Design review of the part shown in the three views and the two pictorial views. Dimensions are in mm from the part's minimum x, y and z. Give positions to 0.01 mm unless a question says otherwise; leave off trailing zeros. Loops run counter-clockwise (first coordinate to the right, second up) from the corner with the lowest first, then second, coordinate; pieces in that order, holes last. Notation, with made-up numbers: (-20, 11) -> (29, 11) arc R19 cw to (29, 48) -> close; hole circle Ø5 at (-30, 6). An arc over 180 degrees is marked (long way). Answer as CSV lines item,"result".
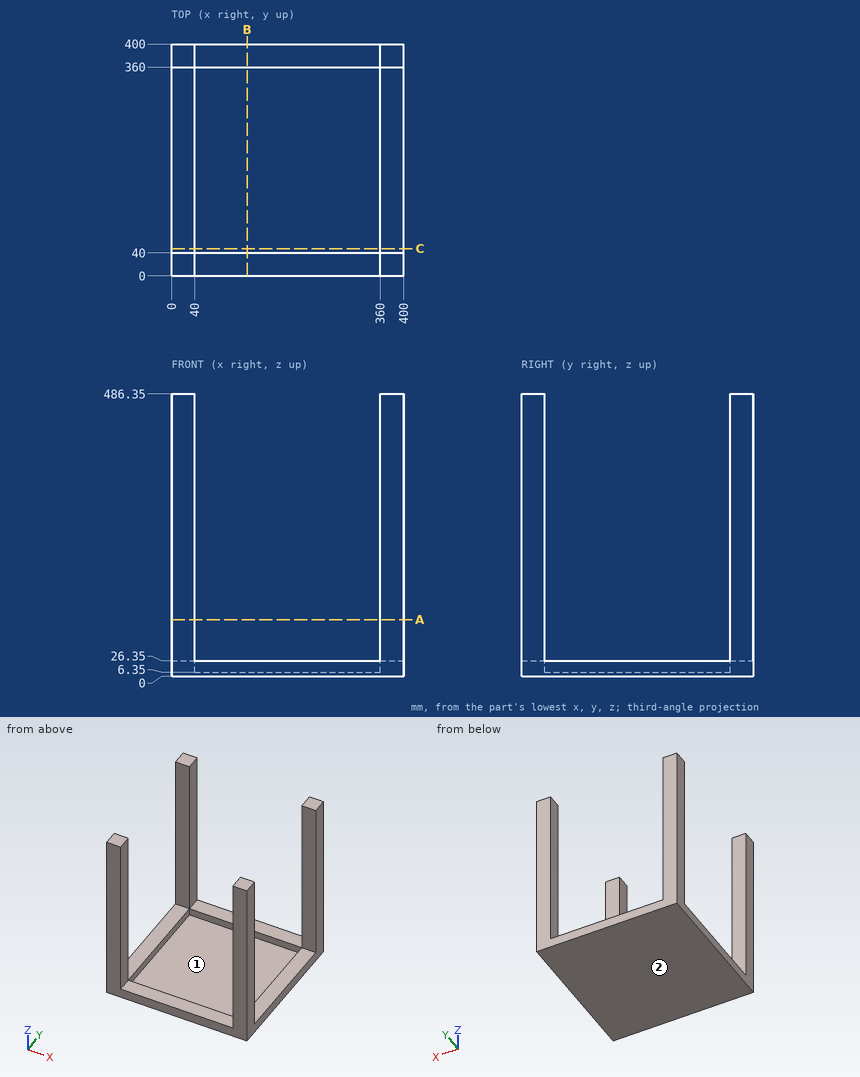
Q1. We need section A-A, the plane z = 97. State the section outline as (x, y) points.
Filled sheet:
outline,"(0, 0) -> (40, 0) -> (40, 40) -> (0, 40) -> close; (0, 360) -> (40, 360) -> (40, 400) -> (0, 400) -> close; (360, 0) -> (400, 0) -> (400, 40) -> (360, 40) -> close; (360, 360) -> (400, 360) -> (400, 400) -> (360, 400) -> close"
Q2. Clearance check with a flat-ended pin moving along its axis: pin 1 Ø8 at (x, y) = (143, 346.5) entering from +Z. State where the tip first meets the part, or that it passes through.
Filled sheet:
pin 1,"stops at z = 6.35"
Q3. To check wall thickness, follow probe 1 along Y at (x, z) = (38.5, 199); probe 2 along Z at (x, y) = (50.5, 90). State the ranges of each line that lie inside material, in increasing order. Write a range as from..to.
Filled sheet:
probe 1,"y = 0..40, 360..400"
probe 2,"z = 0..6.35"
Q4. The part is to be moulded in two halves that separate along Y. For the marked faces 1 and 2, say which applies: pulls with the +Y half, pulls with the -Y half, needs draft (parallel to the pull), parting line crosses it, or undercut.
Filled sheet:
face 1,"undercut"
face 2,"needs draft"
Q5. We need section B-B, the plane x = 130.5. State the section outline as (y, z) points, and give its area (3 significant figures).
Filled sheet:
outline,"(0, 0) -> (400, 0) -> (400, 26.35) -> (360, 26.35) -> (360, 6.35) -> (40, 6.35) -> (40, 26.35) -> (0, 26.35) -> close"
area,"4,140 mm^2"
